Input: part model. Units: mm. Frame: model coordinates. Face numbers are marked on the shaded views. A direction names the side the tool comes from. Coordinates: 2 decimals unless noted, no trailing zeros. Loops run counter-clockwise (first coordinate to the right, second up) from the corner with the lowest first, then second, coordinate; pieces in that order, holes last.
Item 1: Section A-A on x = 0. Return loops of the section in (y, z).
Item 2: Contact query for flat-ended pins moving along their axis: P1, Ø1, axis at x = 0, z = -6.5, coming from the +Y side; P2, Ø2, axis at y = 12.5, z = -2, coming from the -X side; P3, Ø2, axis at y = 16, z = -7, coming from the +X side. Output: stop coordinate, or through.
Item 3: Section B-B on z = -3. Return loops of the section in (x, y).
Item 4: Reachability of the marked faces 1 and 2 from +Z, -Z, +X, -X, +Y, -Y: full face, straight path, thin tool, end or side. Return the list, or none.
Item 5: Section C-C on y = 11.5. Return loops of the section in (x, z).
Item 6: Ray query, line 1 along X through (y, z) = (19.75, -1.25); line 2 along X through (y, z) = (16.5, -6.75); line 3 along X through (y, z) = (10.5, -0.5). Return the intervals inside material, ascending.
Item 7: Section D-D on z = -0.5. Return loops of the section in (x, y).
```python
from build123d import *

# Parameters (mm, degrees)
BOSS_EXTRU_3_DEPTH      = 16
BOSS_EXTRU_4_REACH      = 27.471
BOSS_EXTRU_4_END_RADIUS = 5
ESQUISSE4_W             = 2
ESQUISSE4_H             = 2


with BuildPart() as part:
    # Esquisse3 → Boss.-Extru.3 (new body)
    with BuildSketch(Plane(origin=(0, 7.659672056, 0), x_dir=(-1, 0, 0), z_dir=(0, 1, 0))):
        with BuildLine():
            Line((-4, 0), (-5, 0))
            ThreePointArc((-5, 0), (0, -5), (5, 0))
            Line((5, 0), (4, 0))
            ThreePointArc((4, 0), (0, -4), (-4, 0))
        make_face()
    extrude(amount=BOSS_EXTRU_3_DEPTH)

    # Boss.-Extru.4: up to this cylinder (the profile starts outside it)
    boss_extru_4_end = Plane(origin=(0, 15.659672, 0), z_dir=(0, -1, 0)) * Cylinder(BOSS_EXTRU_4_END_RADIUS, 65.942, mode=Mode.PRIVATE)
    # Esquisse4 → Boss.-Extru.4 (add, up to the surface)
    with BuildSketch(Plane.XY.offset(-8), mode=Mode.PRIVATE) as boss_extru_4_sk1:
        with Locations((0, 15.659672056)):
            Rectangle(ESQUISSE4_W, ESQUISSE4_H)
    boss_extru_4_tool1 = extrude(boss_extru_4_sk1.sketch, amount=BOSS_EXTRU_4_REACH, mode=Mode.PRIVATE) - boss_extru_4_end
    add(boss_extru_4_tool1.solids().sort_by_distance((0, 15.659672, -8))[0])


solid = part.part
```
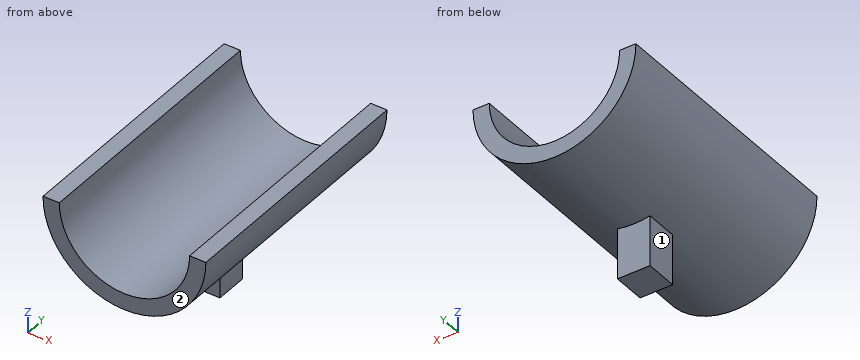
Results found:
1. outline: (7.66, -5) - (14.66, -5) - (14.66, -8) - (16.66, -8) - (16.66, -5) - (23.66, -5) - (23.66, -4) - (7.66, -4) - close
2. P1: stops at y = 16.66
2. P2: stops at x = -4.9
2. P3: stops at x = 1
3. outline: (-4, 7.66) - (-2.65, 7.66) - (-2.65, 23.66) - (-4, 23.66) - close; (2.65, 7.66) - (4, 7.66) - (4, 23.66) - (2.65, 23.66) - close
4. face 1: -Z, -X, +Y, -Y
4. face 2: +Z, -Z, +X, -X, -Y
5. outline: (-5, 0) arc R5 ccw to (5, 0) - (4, 0) arc R4 cw to (-4, 0) - close
6. line 1: x = -4.84 to -3.8, 3.8 to 4.84
6. line 2: x = -1 to 1
6. line 3: x = -4.97 to -3.97, 3.97 to 4.97
7. outline: (-4.97, 7.66) - (-3.97, 7.66) - (-3.97, 23.66) - (-4.97, 23.66) - close; (3.97, 7.66) - (4.97, 7.66) - (4.97, 23.66) - (3.97, 23.66) - close
